```python
from build123d import *

# Parameters (mm, degrees)
SKETCH1_W           = 30
SKETCH1_H           = 34
BOSS_EXTRUDE1_DEPTH = 3
SKETCH3_W           = 27.5
SKETCH3_H           = 31.5
BOSS_EXTRUDE2_DEPTH = 25.5
FILLET1_R           = 3
BOSS_EXTRUDE3_DEPTH = 5
SKETCH5_OUTSIDE_W   = 42.712
SKETCH5_OUTSIDE_H   = 46.712
SKETCH5_OUTSIDE_W_2 = 1.709929724
SKETCH5_OUTSIDE_H_2 = 8.726730488
CUT_EXTRUDE1_DEPTH  = 8


with BuildPart() as part:
    # Sketch1 → Boss-Extrude1 (new body)
    with BuildSketch(Plane.XY):
        Rectangle(SKETCH1_W, SKETCH1_H)
    extrude(amount=-BOSS_EXTRUDE1_DEPTH)

    # Sketch3 → Boss-Extrude2 (add)
    with BuildSketch(Plane.XY):
        Rectangle(SKETCH3_W, SKETCH3_H)
    extrude(amount=BOSS_EXTRUDE2_DEPTH)

    # Fillet1
    fillet1_edges = [part.edges().sort_by_distance(p)[0] for p in [
        (13.75, -15.75, 12.75),
        (13.75, 15.75, 12.75),
        (-13.75, 15.75, 12.75),
        (-13.75, -15.75, 12.75),
        (15, -17, -1.5),
        (-15, -17, -1.5),
        (-15, 17, -1.5),
        (15, 17, -1.5),
    ]]
    fillet(fillet1_edges, radius=FILLET1_R)

    # Sketch4 → Boss-Extrude3 (add, symmetric)
    with BuildSketch(Plane(origin=(0, 0, 0), x_dir=(0, 0, -1), z_dir=(1, 0, 0))):
        with BuildLine():
            Line((-2.5, 15.75), (-2.5, 16.5))
            ThreePointArc((-2.5, 16.5), (-2.676424395, 16.881180834), (-3.081195313, 16.993363275))
            Line((-3.081195313, 16.993363275), (-10.636185348, 15.75))
            Line((-10.636185348, 15.75), (-2.5, 15.75))
        make_face()
        with BuildLine():
            Line((-2.5, -15.75), (-10.636185348, -15.75))
            Line((-10.636185348, -15.75), (-3.081195313, -16.993363275))
            ThreePointArc((-3.081195313, -16.993363275), (-2.676424395, -16.881180834), (-2.5, -16.5))
            Line((-2.5, -16.5), (-2.5, -15.75))
        make_face()
    extrude(amount=BOSS_EXTRUDE3_DEPTH, both=True)

    # Sketch5 outside → Cut-Extrude1 (cut)
    with BuildSketch(Plane.XY.offset(25.5)):
        Rectangle(SKETCH5_OUTSIDE_W, SKETCH5_OUTSIDE_H)
        with Locations((-9.457120396, 7.933102862)):
            Rectangle(SKETCH5_OUTSIDE_W_2, SKETCH5_OUTSIDE_H_2, mode=Mode.SUBTRACT)
        with Locations((-1.31810636, 10.768093543)):
            Rectangle(SKETCH5_OUTSIDE_W_2, SKETCH5_OUTSIDE_H_2, mode=Mode.SUBTRACT)
        with Locations((-1.31810636, -6.561253842)):
            Rectangle(SKETCH5_OUTSIDE_W_2, SKETCH5_OUTSIDE_H_2, mode=Mode.SUBTRACT)
    extrude(amount=-CUT_EXTRUDE1_DEPTH, mode=Mode.SUBTRACT)


solid = part.part
```
Input: part model. Units: mm. Frame: model coordinates. A direction names the side the tool comes from. Coordinates: 2 decimals unless noted, no trailing zeros. Loops run counter-clockwise (first coordinate to the right, second up) from the corner with the lowest first, then second, coordinate; pieces in that order, holes last.
Q1. Contact query for flat-ended pins moving along their axis: pin 1 (9 mm diameter, centred on y = -7.5, z = 23, fed in from -X); pin 2 (6.5 mm diameter, centred on y = 6, z = 23, fed in from +X); pin 3 (9 mm diameter, centred on y = 10, z = 20.5, fed in from +X). Output: stop coordinate, or through.
Results are:
pin 1: stops at x = -2.17
pin 2: stops at x = -0.46
pin 3: stops at x = 13.75
Q2. Section D-D, the plane z = 4.75. Return the cut outline in (x, y), and give its area (3 significant figures).
Results are:
outline: (-13.75, -12.75) arc R3 ccw to (-10.75, -15.75) - (-5, -15.75) - (-5, -16.72) - (5, -16.72) - (5, -15.75) - (10.75, -15.75) arc R3 ccw to (13.75, -12.75) - (13.75, 12.75) arc R3 ccw to (10.75, 15.75) - (5, 15.75) - (5, 16.72) - (-5, 16.72) - (-5, 15.75) - (-10.75, 15.75) arc R3 ccw to (-13.75, 12.75) - close
area: 878 mm2
Q3. Section A-A, the plane z = 23.75. Return the cut outline in (x, y).
Results are:
outline: (-10.31, 3.57) - (-8.6, 3.57) - (-8.6, 12.3) - (-10.31, 12.3) - close; (-2.17, -10.92) - (-0.46, -10.92) - (-0.46, -2.2) - (-2.17, -2.2) - close; (-2.17, 6.4) - (-0.46, 6.4) - (-0.46, 15.13) - (-2.17, 15.13) - close
Q4. Mould query, pull axis X, two halves, no side actions, for faces 1 (the flat face through (-15, 0, -1)), 2 (the cylindrical face through (14.1, -16.14, -1.52)), 3 (the flat face through (-2.173, 11, 22)). Classes: +X half, -X half, draft (parallel to the pull), parting line (faces both ways), or undercut.
Results are:
face 1: -X half
face 2: +X half
face 3: undercut
Q5. Section C-C, the plane y = 2. Return the cut outline in (x, z).
Results are:
outline: (-15, -3) - (15, -3) - (15, 0) - (13.75, 0) - (13.75, 17.5) - (-13.75, 17.5) - (-13.75, 0) - (-15, 0) - close
Q6. Set-up query: faces 4 (the flat face through (-10.312, 8, 22)), 5 (the flat face through (-1, 15.131, 22)), 6 (the flat face through (-5, -16, 6)), 7 (the flat face through (-0.463, 11, 22)), 8 (the flat face through (-8.602, 8, 22)). Return all of +Z, -Z, +X, -X, +Y, -Y with unobstructed straight access to the full face (end or side cutting, diameter ignored); none if empty.
Results are:
face 4: +Z, -X, +Y, -Y
face 5: +Z, +X, -X, +Y
face 6: +Z, -X, -Y
face 7: +Z, +X, +Y, -Y
face 8: +Z, +Y, -Y
Q7. Section B-B, the plane x = 6. Return the cut outline in (y, z).
Results are:
outline: (-17, -3) - (17, -3) - (17, 0) - (15.75, 0) - (15.75, 17.5) - (-15.75, 17.5) - (-15.75, 0) - (-17, 0) - close
Q8. Line query: line 1 along X through (y, z) = (10.5, 19.5); line 2 along X through (y, z) = (-1, 14); line 3 along Z through (x, y) = (3, -9.5). Output: solid intervals per line, ascending.
Results are:
line 1: x = -10.31 to -8.6, -2.17 to -0.46
line 2: x = -13.75 to 13.75
line 3: z = -3 to 17.5
